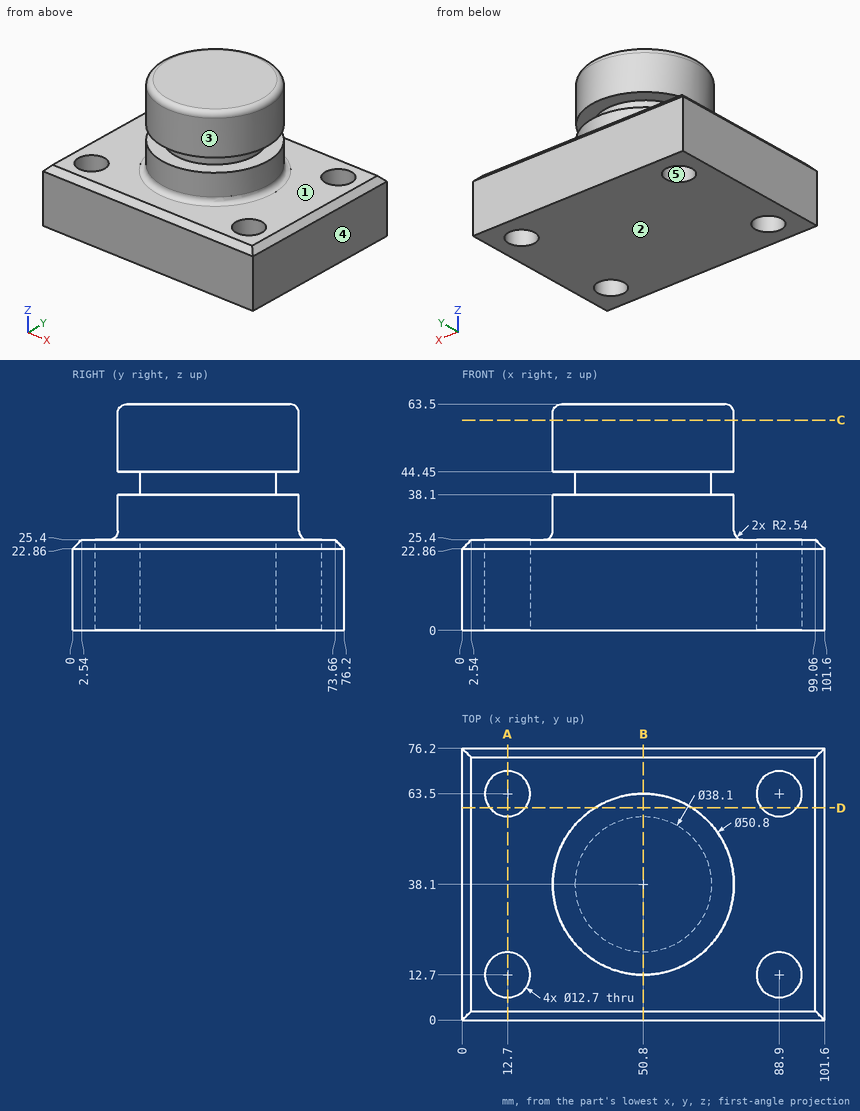
Design review of the part shown in the three views and the two pictorial views. Dimensions are in mm from the part's minimum x, y and z. A direction names the side the tool comes from. Round coordinates to 2 decimals unless told otherwise and drop trailing zeros. Order: outer loops, then holes, each group sorted by start corner. A loop starts at its lowest first (then second) coordinate and runs counter-clockwise, first axis right, second up. Notation, with made-up numbers: (28, -19.75) - (34, -19.75) arc R19 ccw to (34, -0.75) - close; hole circle Ø3 at (88.5, 16). An arc over 180 degrees is marked (long way). Answer in a Markdown table with one row per item.
(1) Mouldability with a two-part tool opening along X and no side actions: class the marked faces 3, 4 and 5 as released by +X, released by -X, zero draft, split by the parting line, or undercut.
Result set:
| item | result |
|---|---|
| face 3 | split by the parting line |
| face 4 | released by +X |
| face 5 | undercut |
(2) For line 1 (X direction, y = 63, z = 19); line 2 (Y direction, x = 88.9, z = 8.25); line 3 (Z direction, x = 19, y = 55.5), list the stretches that pass through material, from the lowest coordinate up. Write a range as from..to.
Result set:
| item | result |
|---|---|
| line 1 | x = 0..6.37, 19.03..82.57, 95.23..101.6 |
| line 2 | y = 0..6.35, 19.05..57.15, 69.85..76.2 |
| line 3 | z = 0..25.4 |
(3) Take a section at A-A on x = 12.7. Write out the cut boundary in (y, z), plus the area to 3 significant figures.
Result set:
| item | result |
|---|---|
| outline | (0, 0) - (6.35, 0) - (6.35, 25.4) - (2.54, 25.4) - (0, 22.86) - close; (19.05, 0) - (57.15, 0) - (57.15, 25.4) - (19.05, 25.4) - close; (69.85, 0) - (76.2, 0) - (76.2, 22.86) - (73.66, 25.4) - (69.85, 25.4) - close |
| area | 1,280 mm2 |
(4) Take a section at C-C on z = 59. Write out the cut boundary in (x, y), plus the area to 3 significant figures.
Result set:
| item | result |
|---|---|
| outline | circle Ø50.8 at (50.8, 38.1) |
| area | 2,030 mm2 |
(5) Take a section at B-B on x = 50.8. Write out the cut boundary in (y, z), plus the area to 3 significant figures.
Result set:
| item | result |
|---|---|
| outline | (0, 0) - (76.2, 0) - (76.2, 22.86) - (73.66, 25.4) - (66.04, 25.4) arc R2.54 cw to (63.5, 27.94) - (63.5, 38.1) - (57.15, 38.1) - (57.15, 44.45) - (63.5, 44.45) - (63.5, 60.96) arc R2.54 ccw to (60.96, 63.5) - (15.24, 63.5) arc R2.54 ccw to (12.7, 60.96) - (12.7, 44.45) - (19.05, 44.45) - (19.05, 38.1) - (12.7, 38.1) - (12.7, 27.94) arc R2.54 cw to (10.16, 25.4) - (2.54, 25.4) - (0, 22.86) - close |
| area | 3,780 mm2 |
(6) Machinability: for the marked faces 1 and 2, which of the approach directions +Z, -Z, +X, -X, +Y, -Y give a long, thin tool a straight path to every point of the face, cutting with its end or side? Answer none if there is none.
Result set:
| item | result |
|---|---|
| face 1 | +Z |
| face 2 | -Z, +X, -X, +Y, -Y |
(7) Clearance check with flat-ended pins moving along their axes: P1, Ø8, axis at x = 86.5, z = 31, coming from the -Y side; P2, Ø10, axis at x = 90, y = 8.5, coming from the +Z side; P3, Ø8, axis at y = 48.5, z = 50.5, coming from the -X side. State where each tip first meets the part, or that it passes through.
Result set:
| item | result |
|---|---|
| P1 | passes through |
| P2 | stops at z = 25.4 |
| P3 | stops at x = 26.22 |
(8) Take a section at D-D on y = 59.5. Count the separate pieces of the cut face and the enclosed holes in it, plus the area to 3 significant figures.
Result set:
| item | result |
|---|---|
| separate pieces | 4 |
| enclosed holes | 0 |
| area | 2,940 mm2 |
